from build123d import *

# Parameters (mm, degrees)
CUT_EXTRUDE1_REACH = 4.5
SKETCH2_R          = 77.5


with BuildPart() as part:
    # Sketch1 → Revolve1 (revolve)
    with BuildSketch(Plane.XY):
        Polygon((0, 0), (77.5, 0), (77.5, 19.5), (85, 19.5), (85, 17), (80, 17), (80, 0), (85, 0), (85, -2.5), (0, -2.5), align=None)
    revolve(axis=Axis((0, -2.5, 0), (0, 1, 0)))

    # Sketch2 → Cut-Extrude1 (cut, up to next)
    with BuildSketch(Plane(origin=(0, 0, 0), x_dir=(1, 0, 0), z_dir=(0, 1, 0)), mode=Mode.PRIVATE) as cut_extrude1_sk1:
        Circle(SKETCH2_R)
    cut_extrude1_tool1 = extrude(cut_extrude1_sk1.sketch, amount=-CUT_EXTRUDE1_REACH, mode=Mode.PRIVATE) & part.part
    add(cut_extrude1_tool1.solids().sort_by_distance((0, 0, 0))[0], mode=Mode.SUBTRACT)


solid = part.part
For this review, take the finished solid that the model builds, in its own axes (mm). A direction names the side the tool comes from. Round coordinates to 2 decimals unless told otherwise and drop trailing zeros. Loops run counter-clockwise (first coordinate to the right, second up) from the corner with the lowest first, then second, coordinate; pieces in that order, holes last. Notation, with made-up numbers: (33.25, 31.25) - (43.25, 31.25) arc R15 ccw to (43.25, 52.25) - close; hole circle Ø4 at (71, 75.25). An arc over 180 degrees is marked (long way). Use one line per item in the form item = value.
1) Tool access review of faces 5 (the face through (63, 17, 50)), 6 (the face through (-67.453, 18.232, 51.721)): name each direction out of +Z, -Z, +X, -X, +Y, -Y from which nothing blocks a thin tool from reaching the whole face with its end or side.
Solutions:
face_5 = none
face_6 = +Y, -Y
2) Mouldability with a two-part tool opening along Y and no side actions: class faces 1 (the face through (69, -2.5, 37)), 2 (the face through (-69, 19.5, 37)), 3 (the face through (-17.34, 8.38, 78.1)), 4 (the face through (-67.453, -1.268, 51.721)) as pulls with the +Y half, pulls with the -Y half, needs draft (parallel to the pull), parting line crosses it, or undercut.
Solutions:
face_1 = pulls with the -Y half
face_2 = pulls with the +Y half
face_3 = undercut
face_4 = needs draft
3) We need section C-C on y = 14.5. Write out the cut boundary in (x, z).
Solutions:
outline = circle Ø160 at (0, 0); hole circle Ø155 at (0, 0)
4) We need section B-B on x = 0. Write out the cut boundary in (y, z), then the cut area to 3 significant figures.
Solutions:
outline = (-2.5, -85) - (0, -85) - (0, -80) - (17, -80) - (17, -85) - (19.5, -85) - (19.5, -77.5) - (-2.5, -77.5) - close; (-2.5, 77.5) - (19.5, 77.5) - (19.5, 85) - (17, 85) - (17, 80) - (0, 80) - (0, 85) - (-2.5, 85) - close
area = 160 mm2
5) Clearance check with flat-ended pins moving along their axes: P1, Ø1, axis at y = 14.5, z = -42, coming from the +X side; P2, Ø12, axis at x = -56.5, y = 5.5, coming from the +Z side; P3, Ø10, axis at y = 0, z = 23, coming from the +X side. State where each tip first meets the part, or that it passes through.
Solutions:
P1 = 68.39
P2 = 65.56
P3 = 83.07
6) We need section A-A on z = 0. Write out the cut boundary in (x, y).
Solutions:
outline = (-85, -2.5) - (-77.5, -2.5) - (-77.5, 19.5) - (-85, 19.5) - (-85, 17) - (-80, 17) - (-80, 0) - (-85, 0) - close; (77.5, -2.5) - (85, -2.5) - (85, 0) - (80, 0) - (80, 17) - (85, 17) - (85, 19.5) - (77.5, 19.5) - close
7) Wall thickness on probe 1 along Z at (x, y) = (0, 9); probe 2 along Y at (x, z) = (-74, 39.5): over which ranges is each line inside the solid? List them lowest first.
Solutions:
probe_1 = -80 to -77.5, 77.5 to 80
probe_2 = -2.5 to 0, 17 to 19.5
